Could you check a few things on this model? Use its own coordinates, in mm. A direction names the side the tool comes from. Give positions to 0.01 mm unless a question says otherwise; leave off trailing zeros. Use a Markdown table: item, result. Add a question column.
Item 1: For faces 1 (the face through (0, 10, 0)), 2 (the face through (-0.9, 6.9, -15.3)), which set-ups out of +Z, -Z, +X, -X, +Y, -Y let a thin tool reach every point of the face, with its end or its side?
Item 2: Suppose I cut it at A-A on x = 0. Count the separate pieces of the cut face and the enclosed holes in it, plus the area to 3 significant figures.
Item 3: If we mould it in two halves opening along Z, with no side actions, what happens to faces 3 (the face through (15.204, 6.916, -0.18)), 4 (the face through (-20.633, 6.916, 15.821)), 5 (the face through (5, 14, 5))? For each: released by +Z, released by -Z, zero draft, split by the parting line, or undercut.
Item 4: If I drill on L1, parallel to Z at x = 0, y = 11.55; L2, parallel to X at y = 6.75, z = 13; L3, parallel to X at y = 3.5, z = -14.5, over which ranges is the centre line in solid material (lowest first)? Write a range as from..to.
Item 5: I'm going to push flat-ended pins straight in: pin 1 Ø4 at (x, y) = (16.5, 7.5) entering from -Z; pin 2 Ø10 at (x, z) = (0, 0) entering from -Y; pin 3 Ø5 at (x, z) = (19.3, 0) entering from +Y; pin 4 Ø5 at (x, y) = (-3.5, 1.5) entering from +Z. Where does each tip first touch, or does it pass through?
from build123d import *

# Parameters (mm, degrees)
SKETCH1_R           = 26
BOSS_EXTRUDE1_DEPTH = 14
SKETCH2_R           = 6.1
CUT_EXTRUDE2_DEPTH  = 4
CUT_EXTRUDE5_START  = 14
SKETCH1_9_R         = 6.25
CUT_EXTRUDE5_DEPTH  = 4
SKETCH1_13_R        = 4.1
CUT_EXTRUDE6_DEPTH  = 8
CUT_EXTRUDE7_START  = 14
SKETCH1_15_R        = 4.1
CUT_EXTRUDE7_DEPTH  = 15
FILLET3_R           = 1
CHAMFER1_SIZE       = 1


with BuildPart() as part:
    # Sketch1 → Boss-Extrude1 (new body)
    with BuildSketch(Plane(origin=(0, 0, 0), x_dir=(1, 0, 0), z_dir=(0, 1, 0))):
        Circle(SKETCH1_R)
    extrude(amount=BOSS_EXTRUDE1_DEPTH)

    # Sketch2 → Cut-Extrude2 (cut)
    with BuildSketch(Plane.XZ):
        Circle(SKETCH2_R)
    extrude(amount=-CUT_EXTRUDE2_DEPTH, mode=Mode.SUBTRACT)

    # Sketch1<9> → Cut-Extrude5 (cut)
    with BuildSketch(Plane(origin=(0, 0, 0), x_dir=(1, 0, 0), z_dir=(0, 1, 0)).offset(CUT_EXTRUDE5_START)):
        Circle(SKETCH1_9_R)
    extrude(amount=-CUT_EXTRUDE5_DEPTH, mode=Mode.SUBTRACT)

    # Sketch1<13> → Cut-Extrude6 (cut)
    with BuildSketch(Plane(origin=(0, 0, 0), x_dir=(1, 0, 0), z_dir=(0, 1, 0))):
        with Locations((-13.647160877, 13.647160877)):
            Circle(SKETCH1_13_R)
        with Locations((0, 19.3)):
            Circle(SKETCH1_13_R)
        with Locations((13.647160877, 13.647160877)):
            Circle(SKETCH1_13_R)
        with Locations((19.3, 0)):
            Circle(SKETCH1_13_R)
        with Locations((13.647160877, -13.647160877)):
            Circle(SKETCH1_13_R)
        with Locations((0, -19.3)):
            Circle(SKETCH1_13_R)
        with Locations((-13.647160877, -13.647160877)):
            Circle(SKETCH1_13_R)
        with Locations((-19.3, 0)):
            Circle(SKETCH1_13_R)
    extrude(amount=CUT_EXTRUDE6_DEPTH, mode=Mode.SUBTRACT)

    # Sketch1<15> → Cut-Extrude7 (cut, through all)
    with BuildSketch(Plane(origin=(0, 0, 0), x_dir=(1, 0, 0), z_dir=(0, 1, 0)).offset(CUT_EXTRUDE7_START)):
        with Locations((-13.647160877, 13.647160877)):
            Circle(SKETCH1_15_R)
        with Locations((0, 19.3)):
            Circle(SKETCH1_15_R)
        with Locations((13.647160877, 13.647160877)):
            Circle(SKETCH1_15_R)
        with Locations((19.3, 0)):
            Circle(SKETCH1_15_R)
        with Locations((13.647160877, -13.647160877)):
            Circle(SKETCH1_15_R)
        with Locations((0, -19.3)):
            Circle(SKETCH1_15_R)
        with Locations((-13.647160877, -13.647160877)):
            Circle(SKETCH1_15_R)
        with Locations((-19.3, 0)):
            Circle(SKETCH1_15_R)
    extrude(amount=-CUT_EXTRUDE7_DEPTH, mode=Mode.SUBTRACT)

    # Fillet3
    fillet3_edges = [part.edges().sort_by_distance(p)[0] for p in [
        (-26, 0, 0),
        (-26, 14, 0),
    ]]
    fillet(fillet3_edges, radius=FILLET3_R)

    # Chamfer1
    chamfer1_edges = [part.edges().sort_by_distance(p)[0] for p in [
        (-17.747160877, 0, 13.647160877),
        (-23.4, 0, 0),
        (-17.747160877, 0, -13.647160877),
        (-4.1, 0, -19.3),
        (9.547160877, 0, -13.647160877),
        (15.2, 0, 0),
        (9.547160877, 0, 13.647160877),
        (-4.1, 0, 19.3),
        (-17.747160877, 14, 13.647160877),
        (-23.4, 14, 0),
        (-17.747160877, 14, -13.647160877),
        (-4.1, 14, -19.3),
        (-4.1, 14, 19.3),
        (9.547160877, 14, 13.647160877),
        (15.2, 14, 0),
        (9.547160877, 14, -13.647160877),
    ]]
    chamfer(chamfer1_edges, length=CHAMFER1_SIZE)


solid = part.part
Findings below:
| question | item | result |
|---|---|---|
| 1 | face 1 | +Y |
| 1 | face 2 | +Y, -Y |
| 2 | separate pieces | 3 |
| 2 | enclosed holes | 0 |
| 2 | area | 395 mm^2 |
| 3 | face 3 | undercut |
| 3 | face 4 | split by the parting line |
| 3 | face 5 | zero draft |
| 4 | L1 | z = -26..-23.4, -15.2..-6.25, 6.25..15.2, 23.4..26 |
| 4 | L2 | x = -22.52..-17.7, -9.6..9.6, 17.7..22.52 |
| 4 | L3 | x = -21.58..-17.66, -9.64..9.64, 17.66..21.58 |
| 5 | pin 1 | stops at z = -21.58 |
| 5 | pin 2 | stops at y = 4 |
| 5 | pin 3 | passes through |
| 5 | pin 4 | stops at z = 25.98 |
